Part model, mm, in its own coordinate system. Coordinates: 2 decimals unless noted, no trailing zeros. Order: outer loops, then holes, each group sorted by start corner. A loop starts at its lowest first (then second) coordinate and runs counter-clockwise, first axis right, second up.
1) Cut at D-D (z = 7). List the corners of the cut face in (x, y).
2) Wall check: L1, parallel to Y at x = 76.2, z = -0.5; L2, parallel to X at y = -81, z = -3; L3, parallel to Y at x = 0, z = -6.25. Give the ranges that are in metal, low to high.
3) Cut at A-A (x = -76.2). List the corners of the cut face in (y, z).
4) Cut at B-B (x = 0). List the corners of the cut face in (y, z), and give its area (3 significant figures).
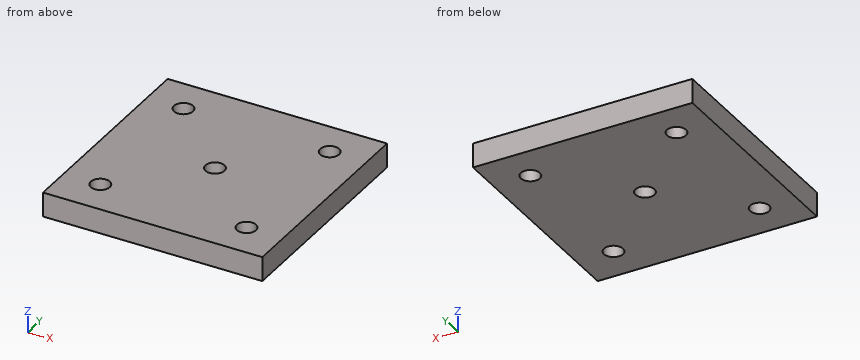
```python
from build123d import *

# Parameters (mm, degrees)
F0_W     = 228.6
F0_H     = 228.6
F1_DEPTH = 12.7
F3_D     = 19.84248
F4_D     = 19.84248


with BuildPart() as f1:
    # F0 (on Top) → F1 (new body, symmetric)
    with BuildSketch(Plane.XY):
        Rectangle(F0_W, F0_H)
    extrude(amount=F1_DEPTH, both=True)

    # F3 (through all)
    with Locations(Plane.XY.offset(12.7)):
        with Locations((-76.2, 76.2), (76.2, 76.2), (-76.2, -76.2), (76.2, -76.2)):
            Hole(F3_D / 2)

    # F4 (through all)
    with Locations(Plane.XY.offset(12.7)):
        with Locations((0, 0)):
            Hole(F4_D / 2)


solid = f1.part
```
Geometry check:
1. outline: (-114.3, -114.3) - (114.3, -114.3) - (114.3, 114.3) - (-114.3, 114.3) - close; hole circle Ø19.84 at (-76.2, -76.2); hole circle Ø19.84 at (-76.2, 76.2); hole circle Ø19.84 at (0, 0); hole circle Ø19.84 at (76.2, -76.2); hole circle Ø19.84 at (76.2, 76.2)
2. L1: y = -114.3 to -86.12, -66.28 to 66.28, 86.12 to 114.3
2. L2: x = -114.3 to -84.88, -67.52 to 67.52, 84.88 to 114.3
2. L3: y = -114.3 to -9.92, 9.92 to 114.3
3. outline: (-114.3, -12.7) - (-86.12, -12.7) - (-86.12, 12.7) - (-114.3, 12.7) - close; (-66.28, -12.7) - (66.28, -12.7) - (66.28, 12.7) - (-66.28, 12.7) - close; (86.12, -12.7) - (114.3, -12.7) - (114.3, 12.7) - (86.12, 12.7) - close
4. outline: (-114.3, -12.7) - (-9.92, -12.7) - (-9.92, 12.7) - (-114.3, 12.7) - close; (9.92, -12.7) - (114.3, -12.7) - (114.3, 12.7) - (9.92, 12.7) - close
4. area: 5,300 mm2
